Part model, mm, in its own coordinate system. A direction names the side the tool comes from. Give positions to 0.01 mm unless a question says otherwise; leave off trailing zeros. Write each loop counter-clockwise with the first axis right and the second up, starting at its lowest first coordinate (ties: lowest second). Pieces come first, ordered by that corner, then holes. Notation, with made-up numbers: M -31,-22 L -22,-22 A24 ccw -22,0 Z; hole C -35.75,61 d3. An arc over 180 degrees is marked long. Answer as CSV lines item,"result". Start each with the question number.
Item 1: Wall check: L1, parallel to Y at x = 69.85, z = -133.5; L2, parallel to X at y = -7, z = -66; L3, parallel to Y at x = 15.5, z = -103.5. Give the ranges that are in metal, low to high. Write a range as from..to.
Item 2: Band-saw the part on C-C, the plane y = -6.35. List the corners of the cut face in (x, z), then the cut area to 3 significant figures.
Item 3: 3-axis set-ups, long thin cutter, end or side, ignore diameter. For faces 1 (the cylindrical face through (9.49, -8.44, -90.14)), 2 (the flat face through (63.5, -6, -90)), 3 (the flat face through (66, 7.62, -154)): which of +Z, -Z, +X, -X, +Y, -Y reach the whole face in a straight line?
Item 4: Band-saw the part on D-D, the plane x = 27. List the corners of the cut face in (y, z), then the cut area to 3 significant figures.
Item 5: Band-saw the part on A-A, the plane x = 69.85. List the corners of the cut face in (y, z), then the cut area to 3 significant figures.
Item 6: Band-saw the part on B-B, the plane z = -17. List the corners of the cut face in (x, y), then the cut area to 3 significant figures.
Item 7: Two-plate mould, pull along X, no slides. Class faces 4 (the flat face through (38, 0, -90)), 5 (the flat face through (76.2, -3, -88)), 6 (the flat face through (0, -2, -90)): +X half, -X half, draft (parallel to the pull), parting line (faces both ways), or undercut.
Item 8: Pin check, flat tips, straight feed: pin 1 (5.5 mm diameter, centred on x = 6.77, y = -6.35, fed in from -Z) (3 decimals); pin 2 (4 mm diameter, centred on x = 20.5, z = -112, fed in from +Y); pin 3 (6.5 mm diameter, centred on y = -3.5, z = -48.5, fed in from -X); pin 4 (4.5 mm diameter, centred on x = 53.01, z = -128.32, fed in from -Y). Stop position of each tip, or through.
from build123d import *

# Parameters (mm, degrees)
SKETCH1_W           = 76.2
SKETCH1_H           = 177.8
BOSS_EXTRUDE1_DEPTH = 7.62
SKETCH4_W           = 12.7
SKETCH4_H           = 177.8
BOSS_EXTRUDE2_DEPTH = 12.7
SKETCH5_R           = 3.429
CUT_EXTRUDE1_DEPTH  = 178.8
SKETCH6_R           = 2.54
SKETCH6_R_2         = 1.778
BOSS_EXTRUDE3_DEPTH = 5.08


with BuildPart() as part:
    # Sketch1 → Boss-Extrude1 (new body)
    with BuildSketch(Plane(origin=(0, 0, 0), x_dir=(1, 0, 0), z_dir=(0, 1, 0))):
        with Locations((38.1, 88.9)):
            Rectangle(SKETCH1_W, SKETCH1_H)
    extrude(amount=BOSS_EXTRUDE1_DEPTH)

    # Sketch4 → Boss-Extrude2 (add)
    with BuildSketch(Plane.XZ):
        with Locations((6.35, -88.9)):
            Rectangle(SKETCH4_W, SKETCH4_H)
        with Locations((69.85, -88.9)):
            Rectangle(SKETCH4_W, SKETCH4_H)
    extrude(amount=BOSS_EXTRUDE2_DEPTH)

    # Sketch5 → Cut-Extrude1 (cut, through all)
    with BuildSketch(Plane(origin=(0, 0, -177.8), x_dir=(-1, 0, 0), z_dir=(0, 0, -1))):
        with Locations((-69.85, -6.35)):
            Circle(SKETCH5_R)
        with Locations((-6.772351806, -6.35)):
            Circle(SKETCH5_R)
    extrude(amount=-CUT_EXTRUDE1_DEPTH, mode=Mode.SUBTRACT)

    # Sketch6 → Boss-Extrude3 (add)
    with BuildSketch(Plane(origin=(0, 7.62, 0), x_dir=(1, 0, 0), z_dir=(0, 1, 0))):
        with Locations((53.0098, 128.3208)):
            Circle(SKETCH6_R)
        with Locations((53.0098, 128.3208)):
            Circle(SKETCH6_R_2, mode=Mode.SUBTRACT)
        with Locations((65.7098, 153.7208)):
            Circle(SKETCH6_R)
        with Locations((65.7098, 153.7208)):
            Circle(SKETCH6_R_2, mode=Mode.SUBTRACT)
    extrude(amount=BOSS_EXTRUDE3_DEPTH)


solid = part.part
Output:
1,L1,"-12.7..-9.78, -2.92..7.62"
1,L2,"0..3.41, 10.14..12.7, 63.5..66.48, 73.22..76.2"
1,L3,"0..7.62"
2,outline,"M 0,-177.8 L 3.34,-177.8 L 3.34,0 L 0,0 Z; M 10.2,-177.8 L 12.7,-177.8 L 12.7,0 L 10.2,0 Z; M 63.5,-177.8 L 66.42,-177.8 L 66.42,0 L 63.5,0 Z; M 73.28,-177.8 L 76.2,-177.8 L 76.2,0 L 73.28,0 Z"
2,area,"2,080 mm²"
3,face 1,"+Z, -Z"
3,face 2,"+Z, -Z, -Y"
3,face 3,"+Y"
4,outline,"M 0,-177.8 L 7.62,-177.8 L 7.62,0 L 0,0 Z"
4,area,"1,350 mm²"
5,outline,"M -12.7,-177.8 L -9.78,-177.8 L -9.78,0 L -12.7,0 Z; M -2.92,-177.8 L 7.62,-177.8 L 7.62,0 L -2.92,0 Z"
5,area,"2,390 mm²"
6,outline,"M 0,-12.7 L 12.7,-12.7 L 12.7,0 L 63.5,0 L 63.5,-12.7 L 76.2,-12.7 L 76.2,7.62 L 0,7.62 Z; hole C 6.77,-6.35 d6.86; hole C 69.85,-6.35 d6.86"
6,area,"829 mm²"
7,face 4,"undercut"
7,face 5,"+X half"
7,face 6,"-X half"
8,pin 1,"through"
8,pin 2,"y = 7.62"
8,pin 3,"x = 0"
8,pin 4,"y = 0"
